Design review of the part shown in the three views and the two pictorial views. Dimensions are in mm from the part's minimum x, y and z. A direction names the side the tool comes from. Round coordinates to 2 decimals unless told otherwise and drop trailing zeros. Order: outer loops, then holes, each group sorted by start corner. A loop starts at its lowest first (then second) coordinate and runs counter-clockwise, first axis right, second up.
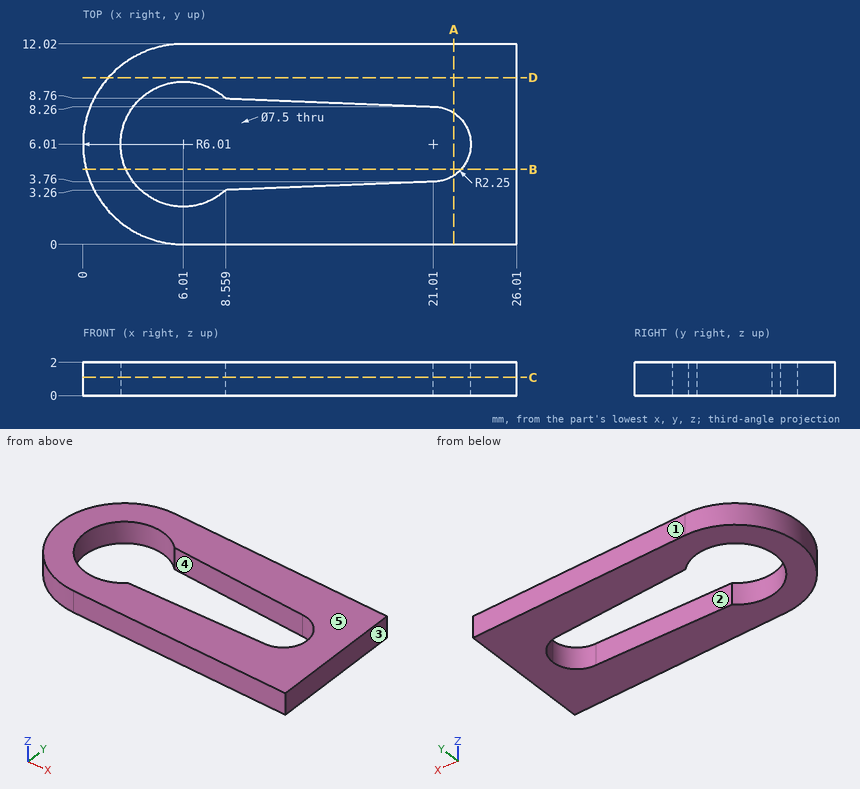
(1) Consider section C-C (z = 1.1). Write out the cut boundary in (x, y).
Data:
outline: (6.01, 0) - (26.01, 0) - (26.01, 12.02) - (6.01, 12.02) arc R6.01 ccw to start; hole (8.56, 3.26) - (21.01, 3.76) arc R2.25 ccw to (21.01, 8.26) - (8.56, 8.76) arc R3.75 ccw (long way) to start
(2) Consider section D-D (y = 10). Write out the cut boundary in (x, z) (1 decimal).
Data:
outline: (1.5, 0) - (26, 0) - (26, 2) - (1.5, 2) - close
(3) For the marked faces 4 and 5, list the 3-axis set-ups (+Z, -Z, +X, -X, +Y, -Y) from which the entire face can be reached by the end or side of a thin tool; tool diameter is ignored.
Data:
face 4: +Z, -Z
face 5: +Z, +X, -X, +Y, -Y
(4) Draft analysis for pull direction Y (two halves, no side actions). For the marked faces 1, 2 and 3, state which applies: pulls with the +Y half, pulls with the -Y half, needs draft (parallel to the pull), parting line crosses it, or undercut.
Data:
face 1: pulls with the +Y half
face 2: undercut
face 3: needs draft
(5) To check wall thickness, follow probe 1 along X at (y, z) = (5.25, 0.7); probe 2 along Y at (x, z) = (5.5, 0.25) (1 decimal); probe 3 along Y at (x, z) = (18.75, 0.2). State the ranges of each line that lie inside material, in increasing order.
Data:
probe 1: x = 0.05 to 2.34, 23.13 to 26.01
probe 2: y = 0 to 2.3, 9.7 to 12
probe 3: y = 0 to 3.67, 8.35 to 12.02
(6) Consider section B-B (y = 4.5). Write out the cut boundary in (x, z).
Data:
outline: (0.19, 0) - (2.58, 0) - (2.58, 2) - (0.19, 2) - close; (22.68, 0) - (26.01, 0) - (26.01, 2) - (22.68, 2) - close
(7) Consider section A-A (x = 22.25). Write out the cut boundary in (y, z).
Data:
outline: (0, 0) - (4.13, 0) - (4.13, 2) - (0, 2) - close; (7.89, 0) - (12.02, 0) - (12.02, 2) - (7.89, 2) - close
